```python
from build123d import *

# Parameters (mm, degrees)
PAD_DEPTH       = 22
THICKNESS_T     = 2
SKETCH001_R     = 5
PAD001_DEPTH    = 3
SKETCH002_R     = 3.6
PAD002_DEPTH    = 6
SKETCH003_R     = 3.6
PAD003_DEPTH    = 6
SKETCH004_R     = 3.6
PAD004_DEPTH    = 6
SKETCH005_R     = 3.6
PAD005_DEPTH    = 6
SKETCH006_R     = 1.6
POCKET_DEPTH    = 11
SKETCH007_R     = 1.6
POCKET001_DEPTH = 11
SKETCH008_R     = 1.6
POCKET002_DEPTH = 11
SKETCH009_R     = 1.6
POCKET003_DEPTH = 11
SKETCH010_R     = 3
POCKET004_DEPTH = 3
POCKET005_DEPTH = 2


with BuildPart() as part:
    # Sketch → Pad (new body)
    with BuildSketch(Plane.XY):
        with BuildLine():
            Line((0, 33), (54, 33))
            ThreePointArc((57, 30), (56.12132, 32.12132), (54, 33))
            Line((57, 30), (57, 0))
            ThreePointArc((54, -3), (56.12132, -2.12132), (57, 0))
            Line((54, -3), (0, -3))
            ThreePointArc((-3, 0), (-2.12132, -2.12132), (0, -3))
            Line((-3, 0), (-3, 30))
            ThreePointArc((0, 33), (-2.12132, 32.12132), (-3, 30))
        make_face()
    extrude(amount=PAD_DEPTH)

    # Thickness
    thickness_openings = [part.faces().sort_by_distance(p)[0] for p in [
        (27, 15, 22),
    ]]
    offset(amount=THICKNESS_T, openings=thickness_openings)

    # Sketch001 → Pad001 (new body)
    with BuildSketch(Plane.XY):
        with Locations((3, 27)):
            Circle(SKETCH001_R)
        with Locations((3, 3)):
            Circle(SKETCH001_R)
        with Locations((27, 27)):
            Circle(SKETCH001_R)
        with Locations((27, 3)):
            Circle(SKETCH001_R)
    extrude(amount=PAD001_DEPTH)

    # Sketch002 → Pad002 (new body)
    with BuildSketch(Plane.XY.offset(3)):
        with Locations((27, 27)):
            Circle(SKETCH002_R)
    extrude(amount=PAD002_DEPTH)

    # Sketch003 → Pad003 (new body)
    with BuildSketch(Plane.XY.offset(3)):
        with Locations((27, 3)):
            Circle(SKETCH003_R)
    extrude(amount=PAD003_DEPTH)

    # Sketch004 → Pad004 (new body)
    with BuildSketch(Plane.XY.offset(3)):
        with Locations((3, 27)):
            Circle(SKETCH004_R)
    extrude(amount=PAD004_DEPTH)

    # Sketch005 → Pad005 (new body)
    with BuildSketch(Plane.XY.offset(3)):
        with Locations((3, 3)):
            Circle(SKETCH005_R)
    extrude(amount=PAD005_DEPTH)

    # Sketch006 → Pocket (cut)
    with BuildSketch(Plane.XY.offset(9)):
        with Locations((27, 27)):
            Circle(SKETCH006_R)
    extrude(amount=-POCKET_DEPTH, mode=Mode.SUBTRACT)

    # Sketch007 → Pocket001 (cut)
    with BuildSketch(Plane.XY.offset(9)):
        with Locations((27, 3)):
            Circle(SKETCH007_R)
    extrude(amount=-POCKET001_DEPTH, mode=Mode.SUBTRACT)

    # Sketch008 → Pocket002 (cut)
    with BuildSketch(Plane.XY.offset(9)):
        with Locations((3, 27)):
            Circle(SKETCH008_R)
    extrude(amount=-POCKET002_DEPTH, mode=Mode.SUBTRACT)

    # Sketch009 → Pocket003 (cut)
    with BuildSketch(Plane.XY.offset(9)):
        with Locations((3, 3)):
            Circle(SKETCH009_R)
    extrude(amount=-POCKET003_DEPTH, mode=Mode.SUBTRACT)

    # Sketch010 → Pocket004 (cut)
    with BuildSketch(Plane(origin=(0, 0, -2), x_dir=(1, 0, 0), z_dir=(0, 0, -1))):
        with Locations((27, -3)):
            Circle(SKETCH010_R)
        with Locations((27, -27)):
            Circle(SKETCH010_R)
        with Locations((3, -3)):
            Circle(SKETCH010_R)
        with Locations((3, -27)):
            Circle(SKETCH010_R)
    extrude(amount=-POCKET004_DEPTH, mode=Mode.SUBTRACT)

    # Sketch011 → Pocket005 (cut)
    with BuildSketch(Plane.YZ.offset(59)):
        with BuildLine():
            Line((12.27, 18), (20.27, 18))
            ThreePointArc((20.77, 17.5), (20.623553, 17.853553), (20.27, 18))
            Line((20.77, 17.5), (20.77, 14.5))
            ThreePointArc((20.27, 14), (20.623553, 14.146447), (20.77, 14.5))
            Line((20.27, 14), (12.27, 14))
            ThreePointArc((11.77, 14.5), (11.916447, 14.146447), (12.27, 14))
            Line((11.77, 14.5), (11.77, 17.5))
            ThreePointArc((12.27, 18), (11.916447, 17.853553), (11.77, 17.5))
        make_face()
    extrude(amount=-POCKET005_DEPTH, mode=Mode.SUBTRACT)


solid = part.part
```
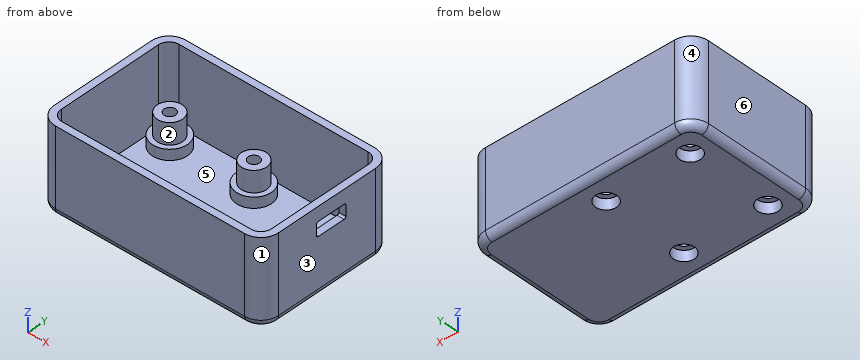
Check sheet for the modelled part. Datum: model origin and axes. Units: mm. Face numbers are marked on the shaded views. A direction names the side the tool comes from. Round coordinates to 2 decimals unless told otherwise and drop trailing zeros. Order: outer loops, then holes, each group sorted by start corner. A loop starts at its lowest first (then second) coordinate and runs counter-clockwise, first axis right, second up. Notation, with made-up numbers: (60, 49.25) - (75, 49.25) arc R27 cw to (75, 88.25) - close; hole circle Ø2 at (70, 75.25). An arc over 180 degrees is marked (long way). Answer as CSV lines item,"result". Start each with the question number.
1) Section check B-B (z = 19.5). Record the cut outline in (x, y).
2) Scan lines: probe 1 along Y at (x, z) = (27, 5.25); probe 2 along Y at (x, z) = (16.5, 10.5); probe 3 along X at (y, z) = (23, 17.5). Record each from-to range of solid material in increasing order.
3) Section check A-A (x = 34). Record the cut outline in (y, z).
4) Draft check along Y on the marked faces 1, 2, 3 and 4. Enter one of: +Y half, -Y half, draft (parallel to the pull), parting line (faces both ways), or undercut.
5) Depth check by flat-ended pin: pin 1 (3 mm diameter, centred on x = 4, y = 1.5, fed in from -Z); pin 2 (8 mm diameter, centred on x = 28.5, y = 2, fed in from +Z); pin 3 (1 mm diameter, centred on x = 58, z = 16, fed in from +Y); pin 4 (0.6 mm diameter, centred on x = 58.5, z = 16.5, fed in from -Y). Enter the tip coordinate at first touch or a pass-through.
6) Section check C-C (y = 3). Give the number of separate pieces and of enclosed holes in the cut face, then the cut area to 3 significant figures.
7) Tool access check on the marked faces 5 and 6. Record the directions out of +Z, -Z, +X, -X, +Y, -Y that give a thin tool (end or side, any length) a straight path to the whole face; none if there is none.
Determined:
1,outline,"(-5, 0) arc R5 ccw to (0, -5) - (54, -5) arc R5 ccw to (59, 0) - (59, 30) arc R5 ccw to (54, 35) - (0, 35) arc R5 ccw to (-5, 30) - close; hole (-3, 0) arc R3 ccw to (0, -3) - (54, -3) arc R3 ccw to (57, 0) - (57, 30) arc R3 ccw to (54, 33) - (0, 33) arc R3 ccw to (-3, 30) - close"
2,probe 1,"-5 to -3, -0.6 to 1.4, 4.6 to 6.6, 23.4 to 25.4, 28.6 to 30.6, 33 to 35"
2,probe 2,"-5 to -3, 33 to 35"
2,probe 3,"-5 to -3, 57 to 59"
3,outline,"(-5, 0) arc R2 ccw to (-3, -2) - (33, -2) arc R2 ccw to (35, 0) - (35, 22) - (33, 22) - (33, 0) - (-3, 0) - (-3, 22) - (-5, 22) - close"
4,face 1,"-Y half"
4,face 2,"undercut"
4,face 3,"draft"
4,face 4,"+Y half"
5,pin 1,"z = -2"
5,pin 2,"z = 9"
5,pin 3,"y = 33.57"
5,pin 4,"y = -2.71"
6,separate pieces,"3"
6,enclosed holes,"0"
6,area,"273 mm^2"
7,face 5,"+Z"
7,face 6,"+Z, -Z, -X, +Y, -Y"
